Model file for the job. Use its own axes, mm. Coordinates: 2 decimals unless noted, no trailing zeros. Loops run counter-clockwise (first coordinate to the right, second up) from the corner with the lowest first, then second, coordinate; pieces in that order, holes last.
from build123d import *

# Parameters (mm, degrees)
BOSS_EXTRUDE1_DEPTH = 3
FILLET1_R           = 1
SKETCH2_R           = 1.7
CUT_EXTRUDE2_DEPTH  = 74.661387443
CUT_EXTRUDE3_DEPTH  = 74.661387443


with BuildPart() as part:
    # Sketch1 → Boss-Extrude1 (new body)
    with BuildSketch(Plane.XY):
        with BuildLine():
            Line((-47, -44), (47, -44))
            ThreePointArc((47, -44), (55.485281374, -40.485281374), (59, -32))
            Line((59, -32), (59, 32))
            ThreePointArc((59, 32), (55.485281374, 40.485281374), (47, 44))
            Line((47, 44), (-47, 44))
            ThreePointArc((-47, 44), (-55.485281374, 40.485281374), (-59, 32))
            Line((-59, 32), (-59, -32))
            ThreePointArc((-59, -32), (-55.485281374, -40.485281374), (-47, -44))
        make_face()
    extrude(amount=BOSS_EXTRUDE1_DEPTH)

    # Fillet1
    fillet1_edges = [part.edges().sort_by_distance(p)[0] for p in [
        (-59, 0, 0),
        (-55.485281374, 40.485281374, 0),
        (0, 44, 0),
        (55.485281374, 40.485281374, 0),
        (59, 0, 0),
        (55.485281374, -40.485281374, 0),
        (0, -44, 0),
        (-55.485281374, -40.485281374, 0),
    ]]
    fillet(fillet1_edges, radius=FILLET1_R)

    # Sketch2 → Cut-Extrude2 (cut, through all)
    with BuildSketch(Plane(origin=(0, 0, 0), x_dir=(-1, 0, 0), z_dir=(0, 0, -1))):
        with Locations((-45, 39)):
            Circle(SKETCH2_R)
        with Locations((-45, -39)):
            Circle(SKETCH2_R)
        with Locations((45, -39)):
            Circle(SKETCH2_R)
        with Locations((45, 39)):
            Circle(SKETCH2_R)
    extrude(amount=-CUT_EXTRUDE2_DEPTH, mode=Mode.SUBTRACT)

    # Sketch6 → Cut-Extrude3 (cut, through all)
    with BuildSketch(Plane(origin=(0, 0, 0), x_dir=(-1, 0, 0), z_dir=(0, 0, -1))):
        with BuildLine():
            Line((-14.5, 1.5), (14.5, 1.5))
            ThreePointArc((14.5, 1.5), (16, 0), (14.5, -1.5))
            Line((14.5, -1.5), (-14.5, -1.5))
            ThreePointArc((-14.5, -1.5), (-16, 0), (-14.5, 1.5))
        make_face()
        with BuildLine():
            Line((-14.5, 7.5), (14.5, 7.5))
            ThreePointArc((14.5, 7.5), (16, 6), (14.5, 4.5))
            Line((14.5, 4.5), (-14.5, 4.5))
            ThreePointArc((-14.5, 4.5), (-16, 6), (-14.5, 7.5))
        make_face()
        with BuildLine():
            Line((-14.5, 13.5), (14.5, 13.5))
            ThreePointArc((14.5, 13.5), (16, 12), (14.5, 10.5))
            Line((14.5, 10.5), (-14.5, 10.5))
            ThreePointArc((-14.5, 10.5), (-16, 12), (-14.5, 13.5))
        make_face()
    extrude(amount=-CUT_EXTRUDE3_DEPTH, mode=Mode.SUBTRACT)


solid = part.part
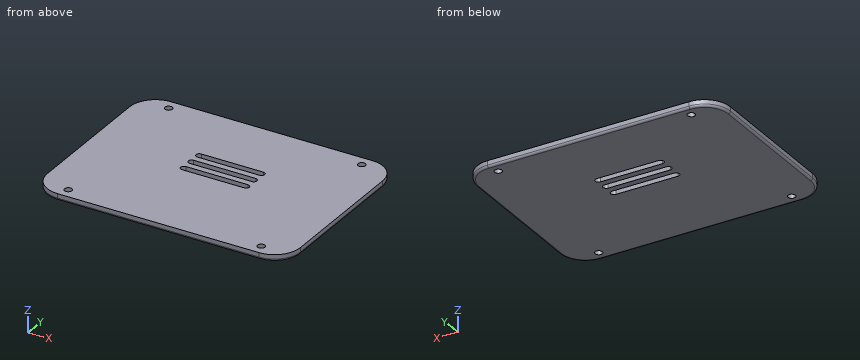
Q1. Drill centre lines: line 1 (Y direction, x = -45, z = 1.35); line 2 (Y direction, x = -45, z = 0.65); line 3 (Y direction, x = -51, z = 2.8). Where is each one in solid material? Low to high.
Answers:
line 1: y = -44 to -40.7, -37.3 to 37.3, 40.7 to 44
line 2: y = -43.94 to -40.7, -37.3 to 37.3, 40.7 to 43.94
line 3: y = -43.31 to 43.31
Q2. Slice it at A-A (y = 12). List the corners of the cut face in (x, z).
Answers:
outline: (-59, 1) arc R1 ccw to (-58, 0) - (-16, 0) - (-16, 3) - (-59, 3) - close; (16, 0) - (58, 0) arc R1 ccw to (59, 1) - (59, 3) - (16, 3) - close
Q3. Slice it at B-B (x = 0.5). List the corners of the cut face in (y, z).
Answers:
outline: (-44, 1) arc R1 ccw to (-43, 0) - (-1.5, 0) - (-1.5, 3) - (-44, 3) - close; (1.5, 0) - (4.5, 0) - (4.5, 3) - (1.5, 3) - close; (7.5, 0) - (10.5, 0) - (10.5, 3) - (7.5, 3) - close; (13.5, 0) - (43, 0) arc R1 ccw to (44, 1) - (44, 3) - (13.5, 3) - close
Q4. Slice it at C-C (x = -45). List the corners of the cut face in (y, z).
Answers:
outline: (-44, 1) arc R1 ccw to (-43, 0) - (-40.7, 0) - (-40.7, 3) - (-44, 3) - close; (-37.3, 0) - (37.3, 0) - (37.3, 3) - (-37.3, 3) - close; (40.7, 0) - (43, 0) arc R1 ccw to (44, 1) - (44, 3) - (40.7, 3) - close
Q5. Slice it at D-D (z = 1.95). List the corners of the cut face in (x, y).
Answers:
outline: (-59, -32) arc R12 ccw to (-47, -44) - (47, -44) arc R12 ccw to (59, -32) - (59, 32) arc R12 ccw to (47, 44) - (-47, 44) arc R12 ccw to (-59, 32) - close; hole circle Ø3.4 at (-45, -39); hole circle Ø3.4 at (-45, 39); hole (-14.5, -1.5) - (14.5, -1.5) arc R1.5 ccw to (14.5, 1.5) - (-14.5, 1.5) arc R1.5 ccw to start; hole (-14.5, 4.5) - (14.5, 4.5) arc R1.5 ccw to (14.5, 7.5) - (-14.5, 7.5) arc R1.5 ccw to start; hole (-14.5, 10.5) - (14.5, 10.5) arc R1.5 ccw to (14.5, 13.5) - (-14.5, 13.5) arc R1.5 ccw to start; hole circle Ø3.4 at (45, -39); hole circle Ø3.4 at (45, 39)
